Geometry: final body of the model. Coordinates: model frame, mm. A direction names the side the tool comes from. Give positions to 0.01 mm unless a question says otherwise; leave off trailing zeros. Loops run counter-clockwise (first coordinate to the right, second up) from the corner with the lowest first, then second, coordinate; pieces in that order, holes last. Notation, with made-up numbers: (37, 11.5) -> (90, 11.5) arc R18 ccw to (90, 17.5) -> close; hole circle Ø11 at (45, -19.75). An arc over 180 degrees is marked (long way). Answer in a Markdown table with one row per item. Add a question column.
1) Line query: line 1 (X direction, y = 0.8, z = -8); line 2 (Y direction, x = -11, z = -17); line 3 (X direction, y = 1.55, z = 13). Output: solid intervals per line, ascending. Write a range as from..to.
2) Section query C-C (x = 11). Give the number of separate pieces and of enclosed holes in the cut face, plus the area to 3 significant figures.
3) Draft query along Y for faces 4 (the cylindrical face through (-28.4, 21.43, 10.99)), 5 (the cylindrical face through (10, 1, -1)), 6 (the cylindrical face through (19, 12, -17)). Return one class per face: +Y half, -Y half, draft (parallel to the pull), parting line (faces both ways), or undercut.
4) Section query A-A (y = 10). Return the cut outline in (x, z), plus the area to 3 significant figures.
5) First-contact query: P1, Ø2.5, axis at x = 11, y = 12, coming from the +Z side; P2, Ø10, axis at x = -18, y = 18, coming from the +Z side; P3, Ø1, axis at x = -25, z = 11, coming from the +Y side. Flat tips, straight axial feed; report the tip coordinate or a pass-through.
6) Section query D-D (y = 16). Return the cut outline in (x, z).
7) Access query for faces 1 (the flat face through (21, 10, 11)), 2 (the flat face through (25, 12, 10)), 3 (the flat face through (21, 9.3, -16.4)). Directions: +Z, -Z, +X, -X, +Y, -Y. A direction counts if a zero-diameter tool reaches every point of the face in a straight line with its end or side. Return the directions, or none.
8) Section query B-B (z = -8). Return the cut outline in (x, y).
```python
from build123d import *

# Parameters (mm, degrees)
SKETCH_1_R              = 4
SKETCH_1_R_2            = 1
SKETCH_1_R_3            = 2
EXTRUDE_1_DEPTH         = 2
FILLET_1_R              = 2
FILLET_2_R              = 2
FILLET_3_R              = 2
FILLET_4_R              = 2
SKETCH_2_W              = 42
SKETCH_2_H              = 24
SKETCH_2_R              = 1
EXTRUDE_2_DEPTH         = 2
FILLET_5_R              = 2
FILLET_6_R              = 2
FILLET_7_R              = 2
SKETCH_3_W              = 8
SKETCH_3_H              = 22
SKETCH_3_R              = 2
EXTRUDE_3_DEPTH         = 2
FILLET_8_R              = 2
FILLET_9_R              = 2
FILLET_10_R             = 2
FILLET_10_OF_MIRROR_3_R = 2
FILLET_11_R             = 2
FILLET_12_R             = 2


with BuildPart() as part:
    # 草图1 → 凸台-拉伸1 (new body)
    with BuildSketch(Plane(origin=(0, 0, 0), x_dir=(1, 0, 0), z_dir=(0, 1, 0))):
        Polygon((-29, 10), (-21, 10), (-21, 18), (21, 18), (21, 10), (29, 10), (29, -12), (21, -12), (21, -8), (19, -8), (19, -12), (19, -18), (-19, -18), (-19, -12), (-19, -8), (-21, -8), (-21, -12), (-29, -12), align=None)
        with Locations(Location((-11, -6, 0), (0, 0, 270))):
            Circle(SKETCH_1_R, mode=Mode.SUBTRACT)
        with Locations(Location((-11, 1, 0), (0, 0, 270))):
            Circle(SKETCH_1_R_2, mode=Mode.SUBTRACT)
        with Locations(Location((0, 8, 0), (0, 0, 270))):
            Circle(SKETCH_1_R, mode=Mode.SUBTRACT)
        with Locations(Location((0, 15, 0), (0, 0, 270))):
            Circle(SKETCH_1_R_2, mode=Mode.SUBTRACT)
        with Locations(Location((7, 8, 0), (0, 0, 270))):
            Circle(SKETCH_1_R_2, mode=Mode.SUBTRACT)
        with Locations(Location((0, 1, 0), (0, 0, 270))):
            Circle(SKETCH_1_R_2, mode=Mode.SUBTRACT)
        with Locations(Location((-7, 8, 0), (0, 0, 270))):
            Circle(SKETCH_1_R_2, mode=Mode.SUBTRACT)
        with Locations(Location((-4, -6, 0), (0, 0, 270))):
            Circle(SKETCH_1_R_2, mode=Mode.SUBTRACT)
        with Locations(Location((-11, -13, 0), (0, 0, 270))):
            Circle(SKETCH_1_R_2, mode=Mode.SUBTRACT)
        with Locations(Location((-18, -6, 0), (0, 0, 270))):
            Circle(SKETCH_1_R_2, mode=Mode.SUBTRACT)
        with Locations(Location((18, -6, 0), (0, 0, 90))):
            Circle(SKETCH_1_R_2, mode=Mode.SUBTRACT)
        with Locations(Location((11, -13, 0), (0, 0, 90))):
            Circle(SKETCH_1_R_2, mode=Mode.SUBTRACT)
        with Locations(Location((4, -6, 0), (0, 0, 90))):
            Circle(SKETCH_1_R_2, mode=Mode.SUBTRACT)
        with Locations(Location((11, -6, 0), (0, 0, 90))):
            Circle(SKETCH_1_R, mode=Mode.SUBTRACT)
        with Locations(Location((11, 1, 0), (0, 0, 90))):
            Circle(SKETCH_1_R_2, mode=Mode.SUBTRACT)
        with Locations(Location((24, -6, 0), (0, 0, 270))):
            Circle(SKETCH_1_R_3, mode=Mode.SUBTRACT)
        with Locations(Location((24, 4, 0), (0, 0, 270))):
            Circle(SKETCH_1_R_3, mode=Mode.SUBTRACT)
        with Locations(Location((-24, -6, 0), (0, 0, 90))):
            Circle(SKETCH_1_R_3, mode=Mode.SUBTRACT)
        with Locations(Location((-24, 4, 0), (0, 0, 90))):
            Circle(SKETCH_1_R_3, mode=Mode.SUBTRACT)
    extrude_1 = extrude(amount=EXTRUDE_1_DEPTH)

    # 圆角1
    fillet_1_edges = [part.edges().sort_by_distance(p)[0] for p in [
        (29, 1, -10),
    ]]
    fillet(fillet_1_edges, radius=FILLET_1_R)

    # 圆角2
    fillet_2_edges = [part.edges().sort_by_distance(p)[0] for p in [
        (-29, 1, -10),
    ]]
    fillet(fillet_2_edges, radius=FILLET_2_R)

    # 圆角3
    fillet_3_edges = [part.edges().sort_by_distance(p)[0] for p in [
        (-19, 1, 18),
    ]]
    fillet(fillet_3_edges, radius=FILLET_3_R)

    # 圆角4
    fillet_4_edges = [part.edges().sort_by_distance(p)[0] for p in [
        (19, 1, 18),
    ]]
    fillet(fillet_4_edges, radius=FILLET_4_R)

    # 草图2 → 凸台-拉伸2 (add)
    with BuildSketch(Plane(origin=(0, 0, -18), x_dir=(-1, 0, 0), z_dir=(0, 0, -1))):
        with Locations((0, 12)):
            Rectangle(SKETCH_2_W, SKETCH_2_H)
        with Locations((11, 12)):
            Circle(SKETCH_2_R, mode=Mode.SUBTRACT)
        with Locations((11, 19)):
            Circle(SKETCH_2_R, mode=Mode.SUBTRACT)
        with Locations((18, 12)):
            Circle(SKETCH_2_R, mode=Mode.SUBTRACT)
        with Locations((11, 5)):
            Circle(SKETCH_2_R, mode=Mode.SUBTRACT)
        with Locations((4, 12)):
            Circle(SKETCH_2_R, mode=Mode.SUBTRACT)
        with Locations(Location((-18, 12, 0), (0, 0, 180))):
            Circle(SKETCH_2_R, mode=Mode.SUBTRACT)
        with Locations(Location((-11, 19, 0), (0, 0, 180))):
            Circle(SKETCH_2_R, mode=Mode.SUBTRACT)
        with Locations(Location((-11, 5, 0), (0, 0, 180))):
            Circle(SKETCH_2_R, mode=Mode.SUBTRACT)
        with Locations(Location((-4, 12, 0), (0, 0, 180))):
            Circle(SKETCH_2_R, mode=Mode.SUBTRACT)
        with Locations(Location((-11, 12, 0), (0, 0, 180))):
            Circle(SKETCH_2_R, mode=Mode.SUBTRACT)
    extrude(amount=-EXTRUDE_2_DEPTH)

    # 圆角5
    fillet_5_edges = [part.edges().sort_by_distance(p)[0] for p in [
        (21, 24, -17),
    ]]
    fillet(fillet_5_edges, radius=FILLET_5_R)

    # 圆角6
    fillet_6_edges = [part.edges().sort_by_distance(p)[0] for p in [
        (-21, 24, -17),
    ]]
    fillet(fillet_6_edges, radius=FILLET_6_R)

    # 圆角7
    fillet_7_edges = [part.edges().sort_by_distance(p)[0] for p in [
        (0, 0, -18),
    ]]
    fillet(fillet_7_edges, radius=FILLET_7_R - 0.0001)  # a hair under: the kernel refuses the full size

    # 草图3 → 凸台-拉伸3 (add)
    with BuildSketch(Plane.XY.offset(12)):
        with Locations((25, 11)):
            Rectangle(SKETCH_3_W, SKETCH_3_H)
        with Locations((25, 16)):
            Circle(SKETCH_3_R, mode=Mode.SUBTRACT)
        with Locations((25, 6)):
            Circle(SKETCH_3_R, mode=Mode.SUBTRACT)
    extrude_3 = extrude(amount=-EXTRUDE_3_DEPTH)

    # 圆角8
    fillet_8_edges = [part.edges().sort_by_distance(p)[0] for p in [
        (25, 0, 12),
    ]]
    fillet(fillet_8_edges, radius=FILLET_8_R)

    # 圆角9
    fillet_9_edges = [part.edges().sort_by_distance(p)[0] for p in [
        (21, 22, 11),
    ]]
    fillet(fillet_9_edges, radius=FILLET_9_R)

    # 圆角10
    fillet_10_edges = [part.edges().sort_by_distance(p)[0] for p in [
        (29, 22, 11),
    ]]
    fillet(fillet_10_edges, radius=FILLET_10_R)

    # 镜向3: 凸台-拉伸1, 凸台-拉伸3 across plane
    add(extrude_1.mirror(Plane(origin=(0, 0, 0), x_dir=(0, 0, 1), z_dir=(1, 0, 0))))
    add(extrude_3.mirror(Plane(origin=(0, 0, 0), x_dir=(0, 0, 1), z_dir=(1, 0, 0))))

    # 圆角10 of 镜向3
    fillet_10_of_mirror_3_edges = [part.edges().sort_by_distance(p)[0] for p in [
        (-29, 22, 11),
    ]]
    fillet(fillet_10_of_mirror_3_edges, radius=FILLET_10_OF_MIRROR_3_R)

    # 圆角11
    fillet_11_edges = [part.edges().sort_by_distance(p)[0] for p in [
        (-21, 22, 11),
    ]]
    fillet(fillet_11_edges, radius=FILLET_11_R)

    # 圆角12
    fillet_12_edges = [part.edges().sort_by_distance(p)[0] for p in [
        (-25, 0, 12),
    ]]
    fillet(fillet_12_edges, radius=FILLET_12_R)


solid = part.part
```
Evaluation:
| question | item | result |
|---|---|---|
| 1 | line 1 | -29..-8, -6..-4, 4..6, 8..29 |
| 1 | line 2 | 0..4, 6..11, 13..18, 20..24 |
| 1 | line 3 | -19..-12, -10..10, 12..19 |
| 2 | separate pieces | 7 |
| 2 | enclosed holes | 0 |
| 2 | area | 80.0 mm² |
| 3 | face 4 | +Y half |
| 3 | face 5 | draft |
| 3 | face 6 | undercut |
| 4 | outline | (-29, 10) -> (-21, 10) -> (-21, 12) -> (-29, 12) -> close; (-21, -18) -> (21, -18) -> (21, -16) -> (-21, -16) -> close; (21, 10) -> (29, 10) -> (29, 12) -> (21, 12) -> close |
| 4 | area | 116 mm² |
| 5 | P1 | z = -16 |
| 5 | P2 | z = 12 |
| 5 | P3 | y = 22 |
| 6 | outline | (-29, 10) -> (-27, 10) -> (-27, 12) -> (-29, 12) -> close; (-23, 10) -> (-21, 10) -> (-21, 12) -> (-23, 12) -> close; (-21, -18) -> (21, -18) -> (21, -16) -> (-21, -16) -> close; (21, 10) -> (23, 10) -> (23, 12) -> (21, 12) -> close; (27, 10) -> (29, 10) -> (29, 12) -> (27, 12) -> close |
| 7 | face 1 | +Z, +Y, -Y |
| 7 | face 2 | -Z, +X, -X, +Y |
| 7 | face 3 | -Z, +X, +Y, -Y |
| 8 | outline | (-29, 0) -> (-8, 0) -> (-8, 2) -> (-29, 2) -> close; (-6, 0) -> (-4, 0) -> (-4, 2) -> (-6, 2) -> close; (4, 0) -> (6, 0) -> (6, 2) -> (4, 2) -> close; (8, 0) -> (29, 0) -> (29, 2) -> (8, 2) -> close |
